For this review, take the finished solid that the model builds, in its own axes (mm). Face numbers are marked on the shaded views. A direction names the side the tool comes from. Coordinates: 2 decimals unless noted, no trailing zeros. Loops run counter-clockwise (first coordinate to the right, second up) from the corner with the lowest first, then second, coordinate; pieces in that order, holes last. Notation, with made-up numbers: (86.25, 81) - (91.25, 81) arc R23 ccw to (91.25, 106) - close; hole circle Ø3 at (12.25, 16.25). An arc over 180 degrees is marked (long way). Answer as a JSON object with one key per item and string values. Group by question number.
Item 1: Tool access review of the marked faces 1, 2 and 3: name each direction out of +Z, -Z, +X, -X, +Y, -Y from which nothing blocks a thin tool from reaching the whole face with its end or side.
Item 2: Mouldability with a two-part tool opening along X and no side actions: class the marked faces 4, 5 and 6 as released by +X, released by -X, zero draft, split by the parting line, or undercut.
Item 3: To check wall thickness, follow line 1 (Z direction, x = 2, y = 0) (3 decimals); line 2 (Y direction, x = -1, z = 0); line 3 (Y direction, x = 7, z = 0). State the ranges of each line that lie inside material, in increasing order.
Item 4: We need section B-B (x = -7.5). Give the boundary of the cut face in (y, z), then the cut area to 3 significant figures.
Item 5: Clearance check with flat-ended pins moving along their axes: pin 1 (2 mm diameter, centred on x = 12, z = 7.5, fed in from +Y); pin 2 (5 mm diameter, centred on x = 12, z = 2, fed in from +Y); pin 3 (3 mm diameter, centred on y = -8, z = -6, fed in from +X). State where each tip first meets the part, or that it passes through.
Item 6: We need section A-A (x = 0). Give the boundary of the cut face in (y, z) (3 decimals), then the cut area to 3 significant figures.
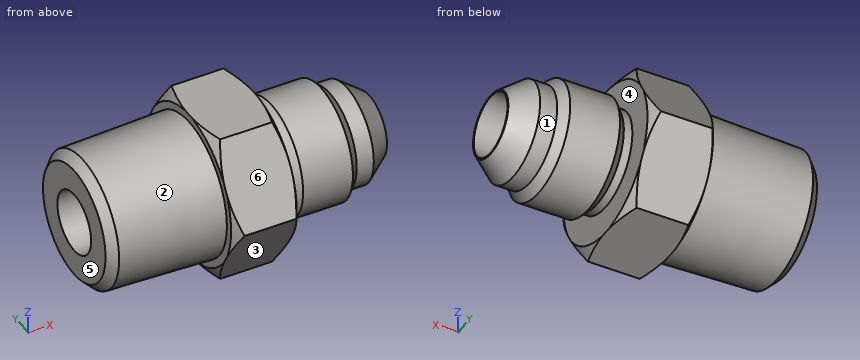
from build123d import *

# Parameters (mm, degrees)
SKETCH6_W           = 36.576
SKETCH6_H           = 7.14375
EXTRUDE1_DEPTH      = 8.128
SKETCH7_W           = 36.576
SKETCH7_H           = 3.81
SKETCH17_R          = 7.14375
CUT_EXTRUDE1_DEPTH  = 14.224
SKETCH19_R          = 8.5725
BOSS_EXTRUDE1_DEPTH = 14.224
BOSS_EXTRUDE1_DRAFT = -1.75
CHAMFER1_SIZE       = 1.058333333
CHAMFER1_SIZE2      = 1.092196811
SKETCH22_R          = 8.5725
BOSS_EXTRUDE3_DEPTH = 14.224
BOSS_EXTRUDE3_DRAFT = -15
SKETCH23_R          = 3.81
CUT_EXTRUDE2_DEPTH  = 14.224


with BuildPart() as part:
    # Sketch6 → Revolve3 (revolve)
    with BuildSketch(Plane.XY, mode=Mode.PRIVATE) as revolve3_sk:
        with Locations((0, 3.571875)):
            Rectangle(SKETCH6_W, SKETCH6_H)
    revolve(revolve3_sk.sketch.rotate(Axis((-18.288, 0, 0), (1, 0, 0)), 90), axis=Axis((-18.288, 0, 0), (1, 0, 0)))

    # Sketch12 → Extrude1 (add)
    with BuildSketch(Plane(origin=(-4.064, 0, 0), x_dir=(0, 0, -1), z_dir=(1, 0, 0))):
        Polygon((0, 10.998522628), (-9.525, 5.499261314), (-9.525, -5.499261314), (0, -10.998522628), (9.525, -5.499261314), (9.525, 5.499261314), align=None)
    extrude(amount=EXTRUDE1_DEPTH)

    # Sketch10 → Cut-Revolve6 (revolve, cut)
    with BuildSketch(Plane.XY, mode=Mode.PRIVATE) as cut_revolve6_sk:
        Polygon((6.165876886, 7.14375), (4.064, 7.14375), (4.064, 6.100206448), (5.122333333, 6.100206448), align=None)
        Polygon((18.288, 7.14375), (12.341385213, 7.14375), (13.384928765, 6.100206448), (15.501595432, 6.100206448), (18.288, 4.0005), align=None)
    revolve(cut_revolve6_sk.sketch.rotate(Axis((-18.288, 0, 0), (1, 0, 0)), 90), axis=Axis((-18.288, 0, 0), (1, 0, 0)), mode=Mode.SUBTRACT)

    # Sketch7 → Cut-Revolve5 (revolve, cut)
    with BuildSketch(Plane.XY):
        with Locations((0, 1.905)):
            Rectangle(SKETCH7_W, SKETCH7_H)
    revolve(axis=Axis((18.288, 0, 0), (-1, 0, 0)), mode=Mode.SUBTRACT)

    # Sketch13 → Cut-Revolve7 (revolve, cut)
    with BuildSketch(Plane.XY):
        Polygon((-4.064, 10.998522628), (-4.064, 9.525), (-3.213261314, 10.998522628), align=None)
        Polygon((3.213261314, 10.998522628), (4.064, 9.525), (4.064, 10.998522628), align=None)
    revolve(axis=Axis((-18.288, 0, 0), (1, 0, 0)), mode=Mode.SUBTRACT)

    # Sketch17 → Cut-Extrude1 (cut)
    with BuildSketch(Plane.ZY.offset(18.288)):
        Circle(SKETCH17_R)
    extrude(amount=-CUT_EXTRUDE1_DEPTH, mode=Mode.SUBTRACT)


with BuildPart() as body_2:
    # Sketch19 → Boss-Extrude1 (with draft: the straight prism first)
    with BuildSketch(Plane(origin=(-4.064, 0, 0), x_dir=(0, 0, -1), z_dir=(1, 0, 0))):
        Circle(SKETCH19_R)
    extrude(amount=-BOSS_EXTRUDE1_DEPTH)
    # Boss-Extrude1: the draft: its side faces are tilted about the plane it starts from
    boss_extrude1_sides = [body_2.faces().sort_by_distance(p)[0] for p in [
        (-11.176, 0, 8.5725),
    ]]
    draft(boss_extrude1_sides, Plane(origin=(-4.064, 0, 0), x_dir=(0, 0, -1), z_dir=(1, 0, 0)), BOSS_EXTRUDE1_DRAFT)

    # Chamfer1
    chamfer1_edges = [body_2.edges().sort_by_distance(p)[0] for p in [
        (-18.288, 0, 8.137917495),
    ]]
    chamfer1_side = [body_2.faces().sort_by_distance(p)[0] for p in [
        (-18.288, 0, 0),
    ]]
    chamfer(chamfer1_edges, length=CHAMFER1_SIZE, length2=CHAMFER1_SIZE2, reference=chamfer1_side[0])


with BuildPart() as boss_extrude3_tool:
    # Sketch22 → Boss-Extrude3 (with draft: the straight prism first)
    with BuildSketch(Plane(origin=(-4.064, 0, 0), x_dir=(0, 0, -1), z_dir=(1, 0, 0))):
        Circle(SKETCH22_R)
    extrude(amount=-BOSS_EXTRUDE3_DEPTH)
    # Boss-Extrude3: the draft: its side faces are tilted about the plane it starts from
    boss_extrude3_sides = [boss_extrude3_tool.faces().sort_by_distance(p)[0] for p in [
        (-11.176, 0, 8.5725),
    ]]
    draft(boss_extrude3_sides, Plane(origin=(-4.064, 0, 0), x_dir=(0, 0, -1), z_dir=(1, 0, 0)), BOSS_EXTRUDE3_DRAFT)


with BuildPart() as body_2_1:
    add(body_2.part)

    # Boss-Extrude3: add boss_extrude3_tool
    add(boss_extrude3_tool.part)

    # Combine1: union part
    add(part.part)

    # Sketch23 → Cut-Extrude2 (cut)
    with BuildSketch(Plane.ZY.offset(18.288)):
        with Locations(Location((0, 0, 0), (0, 0, 90))):
            Circle(SKETCH23_R)
    extrude(amount=-CUT_EXTRUDE2_DEPTH, mode=Mode.SUBTRACT)


solid = body_2_1.part
Check sheet entries:
{
 "1": {"face 1": "+X", "face 2": "-X", "face 3": "-Z, +X, -X, -Y"},
 "2": {"face 4": "undercut", "face 5": "released by -X", "face 6": "zero draft"},
 "3": {"line 1": "z = -9.525 to -3.81, 3.81 to 9.525", "line 2": "y = -11 to -3.81, 3.81 to 11", "line 3": "y = -7.14 to -3.81, 3.81 to 7.14"},
 "4": {"outline": "circle Ø16.94 at (0, 0); hole circle Ø7.62 at (0, 0)", "area": "180 mm2"},
 "5": {"pin 1": "stops at y = 2.96", "pin 2": "stops at y = 7.14", "pin 3": "stops at x = 4.06"},
 "6": {"outline": "(-10.999, 0) - (-5.499, -9.525) - (5.499, -9.525) - (10.999, 0) - (5.499, 9.525) - (-5.499, 9.525) - close; hole circle Ø7.62 at (0, 0)", "area": "269 mm2"}
}
